```python
from build123d import *

# Parameters (mm, degrees)
SKETCH1_W                          = 8.1
SKETCH1_H                          = 11.5
BOSS_EXTRUDE1_DEPTH                = 3.5
SKETCH2_W                          = 6.1
SKETCH2_H                          = 9.5
CUT_EXTRUDE1_DEPTH                 = 2.5
SKETCH3_R                          = 1.5
CUT_EXTRUDE2_DEPTH                 = 2
SKETCH6_R                          = 0.5953125
CUT_EXTRUDE5_DEPTH                 = 2.5
SKETCH7_R                          = 0.79375
CUT_EXTRUDE6_DEPTH                 = 2
SKETCH16_W                         = 8.991857398
SKETCH16_H                         = 1
BACK_CUT_EXTRUDE_DEPTH             = 4
SKETCH17_W                         = 1
SKETCH17_H                         = 6.996497869
SIDE_CUT_EXTRUDE_DEPTH             = 3
SKETCH18_R                         = 0.5
PEG_EXTRUDE_DEPTH                  = 2
FILLET1_R                          = 0.5
TAP_DRILL_SLOT_FOR_0_80_TAP2_D     = 1.19126
TAP_DRILL_SLOT_FOR_0_80_TAP2_DEPTH = 1
TAP_DRILL_SLOT_FOR_0_80_TAP2_TIP   = 0.357890611


with BuildPart() as part:
    # Sketch1 → Boss-Extrude1 (new body)
    with BuildSketch(Plane(origin=(0, 0, 0), x_dir=(1, 0, 0), z_dir=(0, 1, 0))):
        Rectangle(SKETCH1_W, SKETCH1_H)
    extrude(amount=BOSS_EXTRUDE1_DEPTH)

    # Sketch2 → Cut-Extrude1 (cut)
    with BuildSketch(Plane(origin=(0, 3.5, 0), x_dir=(1, 0, 0), z_dir=(0, 1, 0))):
        Rectangle(SKETCH2_W, SKETCH2_H)
    extrude(amount=-CUT_EXTRUDE1_DEPTH, mode=Mode.SUBTRACT)

    # Sketch3 → Cut-Extrude2 (cut, through all)
    with BuildSketch(Plane(origin=(0, 1, 0), x_dir=(1, 0, 0), z_dir=(0, 1, 0))):
        with Locations((0.05, -1.75)):
            Circle(SKETCH3_R)
    extrude(amount=-CUT_EXTRUDE2_DEPTH, mode=Mode.SUBTRACT)

    # Sketch6 → Cut-Extrude5 (cut)
    with BuildSketch(Plane(origin=(0, 3.5, 0), x_dir=(1, 0, 0), z_dir=(0, 1, 0))):
        with Locations((2.629050494, -4.329050494)):
            Circle(SKETCH6_R)
    extrude(amount=-CUT_EXTRUDE5_DEPTH, mode=Mode.SUBTRACT)

    # Sketch7 → Cut-Extrude6 (cut, through all)
    with BuildSketch(Plane(origin=(0, 1, 0), x_dir=(1, 0, 0), z_dir=(0, 1, 0))):
        with Locations((0.05, 1.25)):
            Circle(SKETCH7_R)
        with Locations((-1.825, -3.5)):
            Circle(SKETCH7_R)
        with Locations((1.925, -3.5)):
            Circle(SKETCH7_R)
    extrude(amount=-CUT_EXTRUDE6_DEPTH, mode=Mode.SUBTRACT)

    # Sketch16 → Back-cut-extrude (cut)
    with BuildSketch(Plane.XZ):
        with Locations((-0.234538983, -5.25)):
            Rectangle(SKETCH16_W, SKETCH16_H)
    extrude(amount=-BACK_CUT_EXTRUDE_DEPTH, mode=Mode.SUBTRACT)

    # Sketch17 → Side-cut-extrude (cut)
    with BuildSketch(Plane(origin=(0, 1, 0), x_dir=(1, 0, 0), z_dir=(0, 1, 0))):
        with Locations((-3.55, -1.251751065)):
            Rectangle(SKETCH17_W, SKETCH17_H)
    extrude(amount=SIDE_CUT_EXTRUDE_DEPTH, mode=Mode.SUBTRACT)

    # Sketch18 → Peg-Extrude (add)
    with BuildSketch(Plane(origin=(0, 1, 0), x_dir=(1, 0, 0), z_dir=(0, 1, 0))):
        with Locations((-2.05, 0.75)):
            Circle(SKETCH18_R)
    extrude(amount=PEG_EXTRUDE_DEPTH)

    # Fillet1
    fillet1_edges = [part.edges().sort_by_distance(p)[0] for p in [
        (-2.55, 3, -0.75),
    ]]
    fillet(fillet1_edges, radius=FILLET1_R)

    # Tap Drill Slot for #0-80 Tap2
    with Locations(Plane.ZY.offset(4.05)):
        with Locations((-3.545754268, 2.143662575)):
            Hole(TAP_DRILL_SLOT_FOR_0_80_TAP2_D / 2, depth=TAP_DRILL_SLOT_FOR_0_80_TAP2_DEPTH)
            with Locations((0, 0, -(TAP_DRILL_SLOT_FOR_0_80_TAP2_DEPTH + TAP_DRILL_SLOT_FOR_0_80_TAP2_TIP / 2))):  # 118° drill point
                Cone(0, TAP_DRILL_SLOT_FOR_0_80_TAP2_D / 2, TAP_DRILL_SLOT_FOR_0_80_TAP2_TIP, mode=Mode.SUBTRACT)


solid = part.part
```
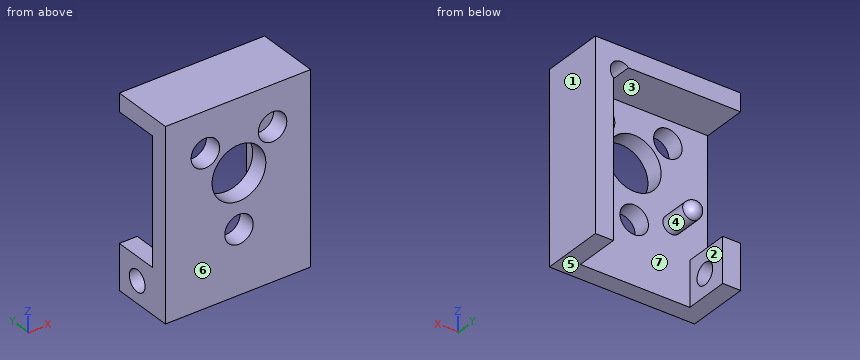
Verification items for the finished model (mm, model axes). Face numbers are marked on the shaded views. A direction names the side the tool comes from. Give positions to 0.01 mm unless a question says otherwise; leave off trailing zeros. Write each loop counter-clockwise with the first axis right and the second up, starting at its lowest first coordinate (ties: lowest second). Pieces come first, ordered by that corner, then holes. Notation, with made-up numbers: (23.25, -0.5) - (78.25, -0.5) arc R19 cw to (78.25, 10.5) - close; hole circle Ø9 at (-8.5, 87). An arc over 180 degrees is marked (long way). Put each result on its own line as item: value.
Q1. Section check C-C on z = 3.5. Record the cut outline in (x, y), and give its area (4 significant figures).
Result:
outline: (-4.05, 0) - (-2.62, 0) - (-2.62, 1) - (-4.05, 1) - close; (-1.03, 0) - (1.13, 0) - (1.13, 1) - (-1.03, 1) - close; (2.72, 0) - (4.05, 0) - (4.05, 3.5) - (3.05, 3.5) - (3.05, 1) - (2.72, 1) - close
area: 7.425 mm2
Q2. Scan lines: probe 1 along Z at (x, y) = (0.05, 0.7); probe 2 along X at (y, z) = (0.55, 3.5); probe 3 along X at (y, z) = (0.65, 1.75). Record each from-to range of solid material in increasing order. Write a range as from..to.
Result:
probe 1: -4.75..-2.04, -0.46..0.25, 3.25..5.75
probe 2: -4.05..-2.62, -1.03..1.13, 2.72..4.05
probe 3: -4.05..-1.45, 1.55..4.05
Q3. Section check D-D on z = 1.75. Record the cut outline in (x, y), and give its area (3 significant figures).
Result:
outline: (-4.05, 0) - (-1.45, 0) - (-1.45, 1) - (-4.05, 1) - close; (1.55, 0) - (4.05, 0) - (4.05, 3.5) - (3.05, 3.5) - (3.05, 1) - (1.55, 1) - close
area: 7.60 mm2
Q4. Set-up check for the marked faces 1, 2 and 3: record each of +Z, -Z, +X, -X, +Y, -Y from which the full face is reachable in a straight line by a thin tool's end or side.
Result:
face 1: +Z, -Z, +X, +Y, -Y
face 2: -Z, +Y
face 3: -X, +Y
Q5. Section check B-B on x = 0.05. Record the cut outline in (y, z), and give its area (3 significant figures).
Result:
outline: (0, -4.75) - (1, -4.75) - (1, -2.04) - (0, -2.04) - close; (0, -0.46) - (1, -0.46) - (1, 0.25) - (0, 0.25) - close; (0, 3.25) - (1, 3.25) - (1, 4.75) - (3.5, 4.75) - (3.5, 5.75) - (0, 5.75) - close
area: 8.41 mm2
Q6. Mould release check, pull along Z, two halves, no side actions. Record for the marked faces 4, 5, 6 and 7: released by +Z, released by -Z, zero draft, split by the parting line, or undercut.
Result:
face 4: undercut
face 5: released by -Z
face 6: zero draft
face 7: undercut
Q7. Depth check by flat-ended pin: P1, Ø2, axis at x = -1.825, z = 3.5, coming from the +Y side. Enter the tip coordinate at first touch or a pass-through.
Result:
P1: y = 1
Q8. Section check A-A on y = 0.85. Count the separate pieces of the cut face and the enclosed holes in it, and give its area (3 significant figures).
Result:
separate pieces: 1
enclosed holes: 4
area: 72.0 mm2
